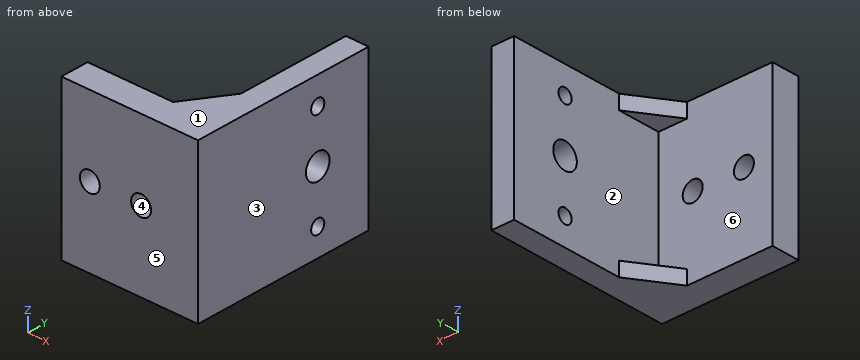
from build123d import *

# Parameters (mm, degrees)
SKETCH1_W           = 48
SKETCH1_H           = 55
BOSS_EXTRUDE1_DEPTH = 10
SKETCH2_W           = 8
SKETCH2_H           = 55
BOSS_EXTRUDE2_DEPTH = 65
SKETCH3_R           = 4.5
CUT_EXTRUDE1_DEPTH  = 65
SKETCH4_R           = 2.5
CUT_EXTRUDE2_DEPTH  = 65
SKETCH5_R           = 3.5
CUT_EXTRUDE4_DEPTH  = 65
BOSS_EXTRUDE3_DEPTH = 5


with BuildPart() as part:
    # Sketch1 → Boss-Extrude1 (new body)
    with BuildSketch(Plane(origin=(0, 0, 0), x_dir=(1, 0, 0), z_dir=(0, 1, 0))):
        Rectangle(SKETCH1_W, SKETCH1_H)
    extrude(amount=BOSS_EXTRUDE1_DEPTH)

    # Sketch2 → Boss-Extrude2 (add)
    with BuildSketch(Plane(origin=(0, 0, 0), x_dir=(1, 0, 0), z_dir=(0, 1, 0))):
        with Locations((20, 0)):
            Rectangle(SKETCH2_W, SKETCH2_H)
    extrude(amount=BOSS_EXTRUDE2_DEPTH)

    # Sketch3 → Cut-Extrude1 (cut)
    with BuildSketch(Plane(origin=(24, 0, 0), x_dir=(0, 0, -1), z_dir=(1, 0, 0))):
        with Locations((0, 45.6)):
            Circle(SKETCH3_R)
    extrude(amount=-CUT_EXTRUDE1_DEPTH, mode=Mode.SUBTRACT)

    # Sketch4 → Cut-Extrude2 (cut)
    with BuildSketch(Plane(origin=(24, 0, 0), x_dir=(0, 0, -1), z_dir=(1, 0, 0))):
        with Locations((-18, 45.6)):
            Circle(SKETCH4_R)
        with Locations((18, 45.6)):
            Circle(SKETCH4_R)
    extrude(amount=-CUT_EXTRUDE2_DEPTH, mode=Mode.SUBTRACT)

    # Sketch5 → Cut-Extrude4 (cut)
    with BuildSketch(Plane(origin=(0, 0, 0), x_dir=(1, 0, 0), z_dir=(0, 1, 0))):
        with Locations((-14, 0)):
            Circle(SKETCH5_R)
        with Locations((4, 0)):
            Circle(SKETCH5_R)
    extrude(amount=CUT_EXTRUDE4_DEPTH, mode=Mode.SUBTRACT)

    # Sketch8 → Boss-Extrude3 (add)
    with BuildSketch(Plane(origin=(0, 0, -27.5), x_dir=(-1, 0, 0), z_dir=(0, 0, -1))):
        Polygon((-16, 25), (-16, 10), (-6, 10), align=None)
    boss_extrude3 = extrude(amount=-BOSS_EXTRUDE3_DEPTH)

    # Mirror1: Boss-Extrude3 across plane
    add(boss_extrude3.mirror(Plane.XY))


solid = part.part
Build history of the part. All positions in model axes, mm. Face numbers are marked on the shaded views. A direction names the side the tool comes from. Give positions to 0.01 mm unless a question says otherwise; leave off trailing zeros. Loops run counter-clockwise (first coordinate to the right, second up) from the corner with the lowest first, then second, coordinate; pieces in that order, holes last. Notation, with made-up numbers: (38, 31.25) - (75, 31.25) arc R14 ccw to (75, 43.25) - close; hole circle Ø11 at (-1, 42.25). An arc over 180 degrees is marked (long way). Write item = value, one per line. Start each with the question number.
1) Pull direction X, two halves, no side cores. Call the marked faces 1, 2, 3 and 4: +X half, -X half, draft (parallel to the pull), parting line (faces both ways), or undercut.
2) Tool access for the marked faces 5 and 6: list every direction of +Z, -Z, +X, -X, +Y, -Y with a clear straight run to the whole face (end or side of a thin tool).
3) Probe probe 1 along X at (y, z) = (6, 0); probe 2 along Z at (x, y) = (-14, 6); probe 3 along Z at (x, y) = (21, 45). List the from-to ranges inside material, lowest first. Write a range as from..to.
4) Drop flat-ended pins along their axis: pin 1 Ø6 at (y, z) = (45.6, -18) entering from -X; pin 2 Ø1.5 at (x, z) = (-7.5, -20) entering from +Y. Give the stop position or say it passes through.
5) Band-saw the part on C-C on y = 45.6. Give the cut face in (x, z).
6) Band-saw the part on B-B on z = -18. Give the cut face in (x, y), plus the area to 3 significant figures.
7) Band-saw the part on A-A on x = -14. Give the cut face in (y, z), plus the area to 3 significant figures.
8) Band-saw the part on D-D on x = 17.5. Give the cut face in (y, z).
Final values:
q1.face_1 = draft
q1.face_2 = -X half
q1.face_3 = +X half
q1.face_4 = undercut
q2.face_5 = +Z, -Z, +X, -X, -Y
q2.face_6 = -X, +Y
q3.probe_1 = -24..-17.5, -10.5..0.5, 7.5..24
q3.probe_2 = -27.5..-3.5, 3.5..27.5
q3.probe_3 = -27.5..-20.43, -15.57..-4.46, 4.46..15.57, 20.43..27.5
q4.pin_1 = 16
q4.pin_2 = 10
q5.outline = (16, -27.5) - (24, -27.5) - (24, -20.5) - (16, -20.5) - close; (16, -15.5) - (24, -15.5) - (24, -4.5) - (16, -4.5) - close; (16, 4.5) - (24, 4.5) - (24, 15.5) - (16, 15.5) - close; (16, 20.5) - (24, 20.5) - (24, 27.5) - (16, 27.5) - close
q6.outline = (-24, 0) - (24, 0) - (24, 43.1) - (16, 43.1) - (16, 10) - (-24, 10) - close; (16, 48.1) - (24, 48.1) - (24, 65) - (16, 65) - close
q6.area = 880 mm²
q7.outline = (0, -27.5) - (10, -27.5) - (10, -3.5) - (0, -3.5) - close; (0, 3.5) - (10, 3.5) - (10, 27.5) - (0, 27.5) - close
q7.area = 480 mm²
q8.outline = (0, -27.5) - (65, -27.5) - (65, 27.5) - (0, 27.5) - close; hole circle Ø9 at (45.6, 0); hole circle Ø5 at (45.6, -18); hole circle Ø5 at (45.6, 18)
